Verification items for the finished model (mm, model axes). Face numbers are marked on the shaded views. A direction names the side the tool comes from. Give positions to 0.01 mm unless a question says otherwise; leave off trailing zeros. Order: outer loops, then holes, each group sorted by start corner. A loop starts at its lowest first (then second) coordinate and runs counter-clockwise, first axis right, second up. Notation, with made-up numbers: M -20,27 L 23,27 A29 cw 23,53 Z; hole C 79.25,-26.5 d4. An arc over 180 degrees is marked long. Answer as a JSON object with one key per item and string values.
```python
from build123d import *

# Parameters (mm, degrees)
BOSS_EXTRUDE2_DEPTH   = 18
F_6_0MM_DOWEL_HOLE4_D = 9
SKETCH16_R            = 8.5
CUT_EXTRUDE1_DEPTH    = 10
SKETCH17_R            = 8.5
CUT_EXTRUDE2_DEPTH    = 45
CUT_EXTRUDE3_DEPTH    = 23.0000001


with BuildPart() as part:
    # Sketch1 → Boss-Extrude2 (new body, symmetric)
    with BuildSketch(Plane.XY):
        with BuildLine():
            Line((18.027756377, 6), (21.027756377, 6))
            Line((21.027756377, 6), (21.027756377, 19))
            Line((21.027756377, 19), (50, 19))
            Line((50, 19), (50, 28))
            Line((50, 28), (25.690465157, 28))
            ThreePointArc((25.690465157, 28), (0, 38), (-25.690465157, 28))
            Line((-25.690465157, 28), (-50, 28))
            Line((-50, 28), (-50, 19))
            Line((-50, 19), (-21.027756377, 19))
            Line((-21.027756377, 19), (-21.027756377, 6))
            Line((-21.027756377, 6), (-18.027756377, 6))
            ThreePointArc((-18.027756377, 6), (0, 19), (18.027756377, 6))
        make_face()
    extrude(amount=BOSS_EXTRUDE2_DEPTH, both=True)

    # Ø6.0mm Dowel Hole4 (through all)
    with Locations(Plane(origin=(0, 28, 0), x_dir=(1, 0, 0), z_dir=(0, 1, 0))):
        with Locations((-31, 0)):
            f_6_0mm_dowel_hole4 = Hole(F_6_0MM_DOWEL_HOLE4_D / 2)

    # Mirror1: Ø6.0mm Dowel Hole4 across plane
    add(f_6_0mm_dowel_hole4.mirror(Plane(origin=(0, 0, 0), x_dir=(0, 0, 1), z_dir=(1, 0, 0))), mode=Mode.SUBTRACT)

    # Sketch16 → Cut-Extrude1 (cut)
    with BuildSketch(Plane(origin=(0, 38, 0), x_dir=(1, 0, 0), z_dir=(0, 1, 0))):
        with Locations((-31, 0)):
            Circle(SKETCH16_R)
    extrude(amount=-CUT_EXTRUDE1_DEPTH, mode=Mode.SUBTRACT)

    # Sketch17 → Cut-Extrude2 (cut)
    with BuildSketch(Plane(origin=(0, 28, 0), x_dir=(1, 0, 0), z_dir=(0, 1, 0))):
        with Locations((31, 0)):
            Circle(SKETCH17_R)
    extrude(amount=CUT_EXTRUDE2_DEPTH, mode=Mode.SUBTRACT)

    # Sketch18 → CBORE for M5 Hex Head Bolt1 (revolve, cut)
    with BuildSketch(Plane(origin=(0, 38, 0), x_dir=(0, 0, 1), z_dir=(1, 0, 0))):
        Polygon((0, 0), (0, 32), (2.5, 32), (2.5, 13.495), (2.995, 13), (3, 13), (3, 0), align=None)
    revolve(axis=Axis((0, 44.35, 0), (0, -1, 0)), mode=Mode.SUBTRACT)

    # Sketch19 → Cut-Extrude3 (cut, through all)
    with BuildSketch(Plane(origin=(0, 28, 0), x_dir=(1, 0, 0), z_dir=(0, 1, 0))):
        with BuildLine():
            Line((-50, 18), (-44.497190923, 18))
            ThreePointArc((-44.497190923, 18), (-48, 0), (-44.497190923, -18))
            Line((-44.497190923, -18), (-50, -18))
            Line((-50, -18), (-50, 18))
        make_face()
    cut_extrude3 = extrude(amount=-CUT_EXTRUDE3_DEPTH, mode=Mode.SUBTRACT)

    # Mirror2: Cut-Extrude3 across plane
    add(cut_extrude3.mirror(Plane(origin=(0, 0, 0), x_dir=(0, 0, 1), z_dir=(1, 0, 0))), mode=Mode.SUBTRACT)


solid = part.part
```
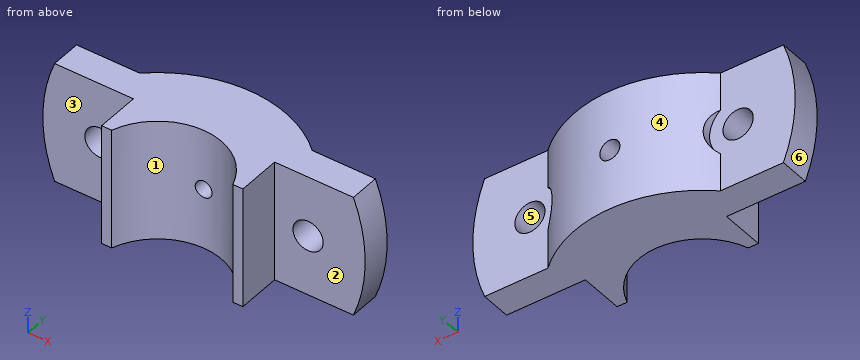
Q1. Tool access check on the marked faces 1, 2 and 3. Record the directions out of +Z, -Z, +X, -X, +Y, -Y that give a thin tool (end or side, any length) a straight path to the whole face; none if there is none.
Resolved:
{"face 1": "+Z, -Z, -Y", "face 2": "+Z, -Z, +X, -Y", "face 3": "+Z, -Z, -X, -Y"}
Q2. Material ranges on L1, parallel to Z at x = 0, y = 20; L2, parallel to Z at x = 31, y = 24.5; L3, parallel to X at y = 21.5, z = -3.5, recorded low to high.
Resolved:
{"L1": "z = -18 to -2.5, 2.5 to 18", "L2": "z = -18 to -4.5, 4.5 to 18", "L3": "x = -47.87 to -33.83, -28.17 to 28.17, 33.83 to 47.87"}
Q3. Section check C-C on y = 17. Record the cut outline in (x, z).
Resolved:
{"outline": "M -21.03,-18 L -8.49,-18 L -8.49,18 L -21.03,18 Z; M 8.49,-18 L 21.03,-18 L 21.03,18 L 8.49,18 Z"}
Q4. Section check B-B on z = 0. Count the separate pieces of the cut face and the enclosed holes in it, then the cut area to 3 significant figures.
Resolved:
{"separate pieces": "4", "enclosed holes": "0", "area": "1,140 mm²"}
Q5. Gauge pin test, flat ends, axial feed: pin 1 Ø5 at (x, z) = (30.5, 12.5) entering from +Y; pin 2 Ø8 at (x, z) = (33, 5) entering from -Y; pin 3 Ø10 at (x, z) = (-27, 7) entering from +Y; pin 4 Ø1.8 at (x, z) = (0.5, -1) entering from +Y. Record the tip position at first contact, or that the pin passes through.
Resolved:
{"pin 1": "stops at y = 28", "pin 2": "stops at y = 19", "pin 3": "stops at y = 30.98", "pin 4": "passes through"}
Q6. Section check A-A on x = 0. Record the cut outline in (y, z) (3 decimals), then the cut area to 3 significant figures.
Resolved:
{"outline": "M 19,-18 L 38,-18 L 38,-3 L 25,-3 L 25,-2.995 L 24.505,-2.5 L 19,-2.5 Z; M 19,2.5 L 24.505,2.5 L 25,2.995 L 25,3 L 38,3 L 38,18 L 19,18 Z", "area": "576 mm²"}
Q7. Section check D-D on x = -31. Record the cut outline in (y, z), then the cut area to 3 significant figures.
Resolved:
{"outline": "M 19,-18 L 28,-18 L 28,-4.5 L 19,-4.5 Z; M 19,4.5 L 28,4.5 L 28,18 L 19,18 Z", "area": "243 mm²"}
Q8. Release check for a two-part mould opening along X. For the marked faces 4, 5 and 6 record: +X half, -X half, draft (parallel to the pull), parting line (faces both ways), or undercut.
Resolved:
{"face 4": "parting line", "face 5": "undercut", "face 6": "-X half"}
